Read the model definition and answer for the solid it produces. Units are mm, in the model's axes. A direction names the side the tool comes from. Give positions to 0.01 mm unless a question says otherwise; leave off trailing zeros. Order: outer loops, then holes, each group sorted by start corner. A loop starts at its lowest first (then second) coordinate and runs counter-clockwise, first axis right, second up. Notation, with made-up numbers: (35, -23) - (82, -23) arc R6 ccw to (82, -12) - close; hole circle Ø2 at (3.25, 58). An arc over 180 degrees is marked (long way). Write each question's results on one line, items separated by ' | '.
from build123d import *

# Parameters (mm, degrees)
SKETCH1_R                                       = 21
SKETCH1_R_2                                     = 1.6
SKETCH1_R_3                                     = 5.5
BOSS_EXTRUDE1_DEPTH                             = 4
SKETCH2_R                                       = 6.5
CUT_EXTRUDE1_DEPTH                              = 1
CSK_FOR_M3_FLAT_HEAD_MACHINE_SCREW1_D           = 3.2
CSK_FOR_M3_FLAT_HEAD_MACHINE_SCREW1_CSINK_D     = 6.3
CSK_FOR_M3_FLAT_HEAD_MACHINE_SCREW1_CSINK_ANGLE = 90


with BuildPart() as part:
    # Sketch1 → Boss-Extrude1 (new body)
    with BuildSketch(Plane.XY):
        Circle(SKETCH1_R)
        with Locations((0, 17.5)):
            Circle(SKETCH1_R_2, mode=Mode.SUBTRACT)
        with Locations((17.5, 0)):
            Circle(SKETCH1_R_2, mode=Mode.SUBTRACT)
        with Locations((0, -17.5)):
            Circle(SKETCH1_R_2, mode=Mode.SUBTRACT)
        with Locations((-17.5, 0)):
            Circle(SKETCH1_R_2, mode=Mode.SUBTRACT)
        Circle(SKETCH1_R_3, mode=Mode.SUBTRACT)
    extrude(amount=BOSS_EXTRUDE1_DEPTH)

    # Sketch2 → Cut-Extrude1 (cut)
    with BuildSketch(Plane.XY.offset(4)):
        Circle(SKETCH2_R)
    extrude(amount=-CUT_EXTRUDE1_DEPTH, mode=Mode.SUBTRACT)

    # CSK for M3 Flat Head Machine Screw1 (through all)
    with Locations(Plane(origin=(0, 0, 0), x_dir=(-1, 0, 0), z_dir=(0, 0, -1))):
        with Locations((17.5, 0), (0, 17.5), (-17.5, 0), (0, -17.5)):
            CounterSinkHole(CSK_FOR_M3_FLAT_HEAD_MACHINE_SCREW1_D / 2, CSK_FOR_M3_FLAT_HEAD_MACHINE_SCREW1_CSINK_D / 2, counter_sink_angle=CSK_FOR_M3_FLAT_HEAD_MACHINE_SCREW1_CSINK_ANGLE)


solid = part.part
(1) Section D-D (z = 0.95) is taken. Give the vertices of the cut face in (x, y).
Conclusion:
outline: circle Ø42 at (0, 0); hole circle Ø4.4 at (-17.5, 0); hole circle Ø11 at (0, 0); hole circle Ø4.4 at (0, -17.5); hole circle Ø4.4 at (0, 17.5); hole circle Ø4.4 at (17.5, 0)
(2) Each of these flat-tipped pins is pushed along its axis until it touches: pin 1 (1.5 mm diameter, centred on y = 9.5, z = 2.5, fed in from +X); pin 2 (3.5 mm diameter, centred on x = -17.5, y = 0, fed in from -Z). Where does it stop, or does it pass through?
Conclusion:
pin 1: x = 19.09 | pin 2: z = 1.4
(3) Section C-C (x = 5) is taken. Give the vertices of the cut face in (y, z).
Conclusion:
outline: (-20.4, 0) - (-2.29, 0) - (-2.29, 3) - (-4.15, 3) - (-4.15, 4) - (-20.4, 4) - close; (2.29, 0) - (20.4, 0) - (20.4, 4) - (4.15, 4) - (4.15, 3) - (2.29, 3) - close
(4) For faces 1 (the face through (4, -4, 0)), 2 (the face through (-5.158, -3.955, 3.507)), determine the directions among +Z, -Z, +X, -X, +Y, -Y from which every point of the face is accessible in a straight line to the end or side of a thin tool.
Conclusion:
face 1: -Z, +X, -X, +Y, -Y | face 2: +Z
(5) Section A-A (x = 0) is taken. Give the vertices of the cut face in (y, z), plus the area to 3 significant figures.
Conclusion:
outline: (-21, 0) - (-20.65, 0) - (-19.1, 1.55) - (-19.1, 4) - (-21, 4) - close; (-15.9, 1.55) - (-14.35, 0) - (-5.5, 0) - (-5.5, 3) - (-6.5, 3) - (-6.5, 4) - (-15.9, 4) - close; (5.5, 0) - (14.35, 0) - (15.9, 1.55) - (15.9, 4) - (6.5, 4) - (6.5, 3) - (5.5, 3) - close; (19.1, 1.55) - (20.65, 0) - (21, 0) - (21, 4) - (19.1, 4) - close | area: 91.6 mm^2
(6) Consider probe 1 along Y at (x, z) = (0, 3.3); probe 2 along Y at (x, z) = (0, 0.85); probe 3 along Y at (x, z) = (18, 0.5). Determine where each line is inside the solid, lowest interval first. Write a range as [from, to].
Conclusion:
probe 1: [-21, -19.1], [-15.9, -6.5], [6.5, 15.9], [19.1, 21] | probe 2: [-21, -19.8], [-15.2, -5.5], [5.5, 15.2], [19.8, 21] | probe 3: [-10.82, -2.6], [2.6, 10.82]
(7) The mould has two halves that part along X. Classify faces 3 (the face through (20.03, 6.31, 1.97)), 4 (the face through (4.4, 5, 4)), 5 (the face through (15.9, 0.07, 2.76)), 6 (the face through (-19.1, 0.07, 2.76)): pulls with the +X half, pulls with the -X half, needs draft (parallel to the pull), parting line crosses it, or undercut.
Conclusion:
face 3: parting line crosses it | face 4: needs draft | face 5: undercut | face 6: undercut
